Read the model definition and answer for the solid it produces. Units are mm, in the model's axes. Coordinates: 2 decimals unless noted, no trailing zeros. Order: outer loops, then holes, each group sorted by start corner. A loop starts at its lowest first (then second) coordinate and runs counter-clockwise, first axis right, second up. Notation, with made-up numbers: (38, -20.75) - (95, -20.75) arc R16 ccw to (95, -7.75) - close; hole circle Ø10 at (-6.5, -24.5). An arc over 180 degrees is marked (long way). Use one line per item in the form item = value.
Autodesk Inventor part; units mm, degrees
ref_plane "YZ Plane" through (0, 0, 0) normal (1, 0, 0) x (0, 1, 0)
ref_plane "XZ Plane" through (0, 0, 0) normal (0, 1, 0) x (-1, 0, 0)
ref_plane "XY Plane" through (0, 0, 0) normal (0, 0, 1) x (1, 0, 0)
sketch "Sketch2" plane through (0, 0, 0) normal (0, 1, 0) x (-1, 0, 0)
  line L0 (-38.1051, 6) -> (13.8564, 36)
  line L1 (-38.1051, 6) -> (-38.1051, -6)
  line L2 (13.8564, -36) -> (-38.1051, -6)
  line L3 (13.8564, -36) -> (24.2487, -30)
  line L4 (24.2487, -30) -> (24.2487, 30)
  line L5 (13.8564, 36) -> (24.2487, 30)
  point P0 (0, 0)
  point P1 (0, 0)
extrude "Extrusion1" add sketch "Sketch2" along normal blind 1.6
properties part number "PCB_Top"
(1) Section A-A, the plane y = 1 is taken. Write down the section's boundary in (x, z), then the cut area to 3 significant figures.
Answer list:
outline = (-24.25, -30) - (-13.86, -36) - (38.11, -6) - (38.11, 6) - (-13.86, 36) - (-24.25, 30) - close
area = 2,870 mm2
(2) Straight lines are drawn through the part: L1, parallel to Z at x = 25.5, y = 0.9; L2, parallel to Z at x = -7.5, y = 0.7; L3, parallel to X at y = 0.3, z = -22.5. For each, find the intervals that lie inside material, in ascending order.
Answer list:
L1 = -13.28 to 13.28
L2 = -32.33 to 32.33
L3 = -24.25 to 9.53
(3) Section C-C, the plane z = -19 is taken. Write down the section's boundary in (x, y), then the cut area to 3 significant figures.
Answer list:
outline = (-24.25, 0) - (15.59, 0) - (15.59, 1.6) - (-24.25, 1.6) - close
area = 63.7 mm2
(4) Section B-B, the plane x = 14 is taken. Write down the section's boundary in (y, z), then the cut area to 3 significant figures.
Answer list:
outline = (0, -19.92) - (1.6, -19.92) - (1.6, 19.92) - (0, 19.92) - close
area = 63.7 mm2
(5) Given pin 1 Ø5 at (x, z) = (30, -14) entering from +Y, flat-ended and moving along its own axis, determine where the tip first touches the part or whether it passes through.
Answer list:
pin_1 = through
